Input: dimensioned drawing with shaded views. Units: mm. Origin: part minimum x, y, z. Give positions to 0.01 mm unless a question says otherwise; leave off trailing zeros. Write each loop counter-clockwise with the first axis right and the second up, starting at its lowest first coordinate (ties: lowest second). Pieces come first, ordered by that corner, then holes.
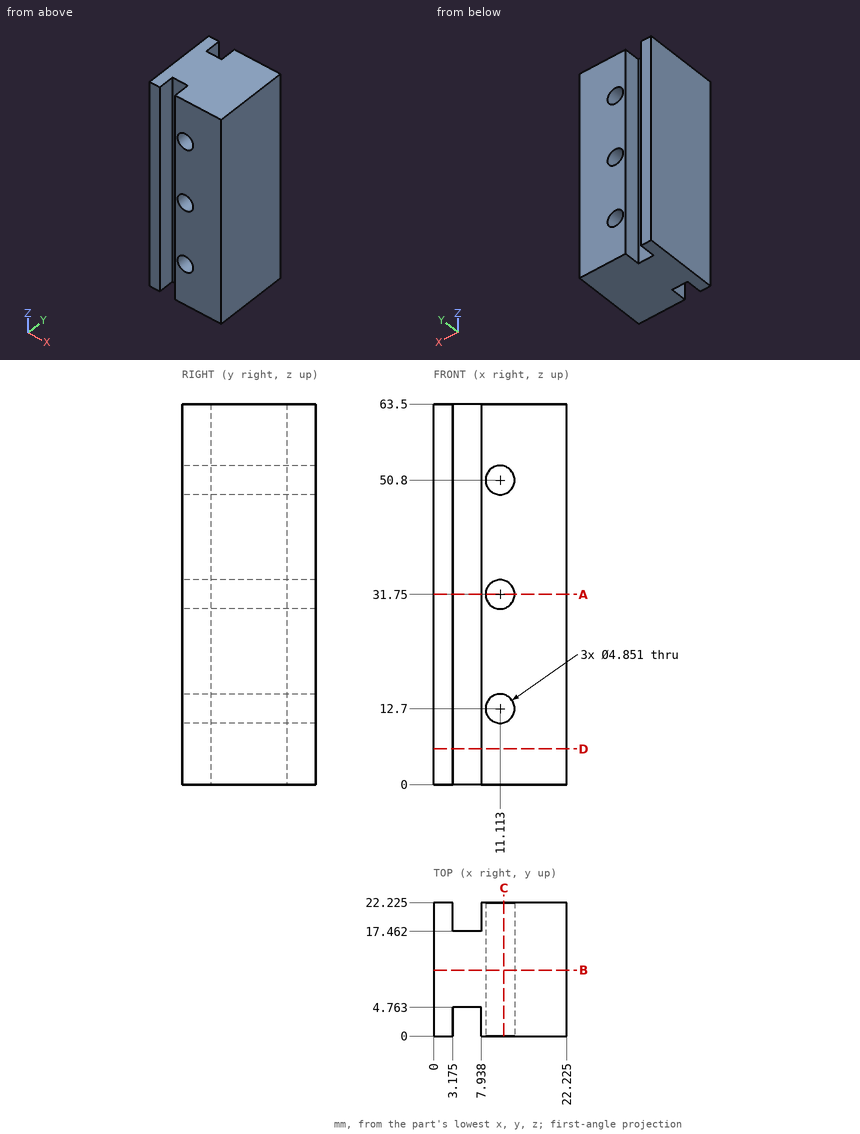
1. Cut plane A-A, the plane z = 31.75. Return the cut outline in (x, y) (1 decimal), then the cut area to 3 significant figures.
2. Line query: L1, parallel to X at y = 8, z = 12.7 (1 decimal); L2, parallel to Z at x = 9.25, y = 5.75 (1 decimal); L3, parallel to Z at x = 9, y = 14.75 (1 decimal). Output: solid intervals per line, ascending.
3. Contact query for flat-ended pins moving along their axis: P1, Ø4, axis at x = 11.11, z = 50.8, coming from the -Y side; P2, Ø3, axis at x = 5, z = 21, coming from the +Y side. Output: stop coordinate, or through.
4. Cut plane B-B, the plane y = 11. State how many separate pieces and enclosed holes the cut face has, then the cut area to 3 significant figures.
5. Cut plane C-C, the plane x = 11.75. Return the cut outline in (y, z) (1 decimal), then the cut area to 3 significant figures.
6. Cut plane D-D, the plane z = 6. Return the cut outline in (x, y) (1 decimal).
Response values:
1. outline: (0, 0) - (3.2, 0) - (3.2, 4.8) - (7.9, 4.8) - (7.9, 0) - (8.7, 0) - (8.7, 22.2) - (7.9, 22.2) - (7.9, 17.5) - (3.2, 17.5) - (3.2, 22.2) - (0, 22.2) - close; (13.5, 0) - (22.2, 0) - (22.2, 22.2) - (13.5, 22.2) - close
1. area: 341 mm2
2. L1: x = 0 to 8.7, 13.5 to 22.2
2. L2: z = 0 to 11.1, 14.3 to 30.2, 33.3 to 49.2, 52.4 to 63.5
2. L3: z = 0 to 11.5, 13.9 to 30.6, 32.9 to 49.6, 52 to 63.5
3. P1: passes through
3. P2: stops at y = 17.46
4. separate pieces: 1
4. enclosed holes: 3
4. area: 1,360 mm2
5. outline: (0, 0) - (22.2, 0) - (22.2, 10.4) - (0, 10.4) - close; (0, 15) - (22.2, 15) - (22.2, 29.4) - (0, 29.4) - close; (0, 34.1) - (22.2, 34.1) - (22.2, 48.5) - (0, 48.5) - close; (0, 53.1) - (22.2, 53.1) - (22.2, 63.5) - (0, 63.5) - close
5. area: 1,100 mm2
6. outline: (0, 0) - (3.2, 0) - (3.2, 4.8) - (7.9, 4.8) - (7.9, 0) - (22.2, 0) - (22.2, 22.2) - (7.9, 22.2) - (7.9, 17.5) - (3.2, 17.5) - (3.2, 22.2) - (0, 22.2) - close
